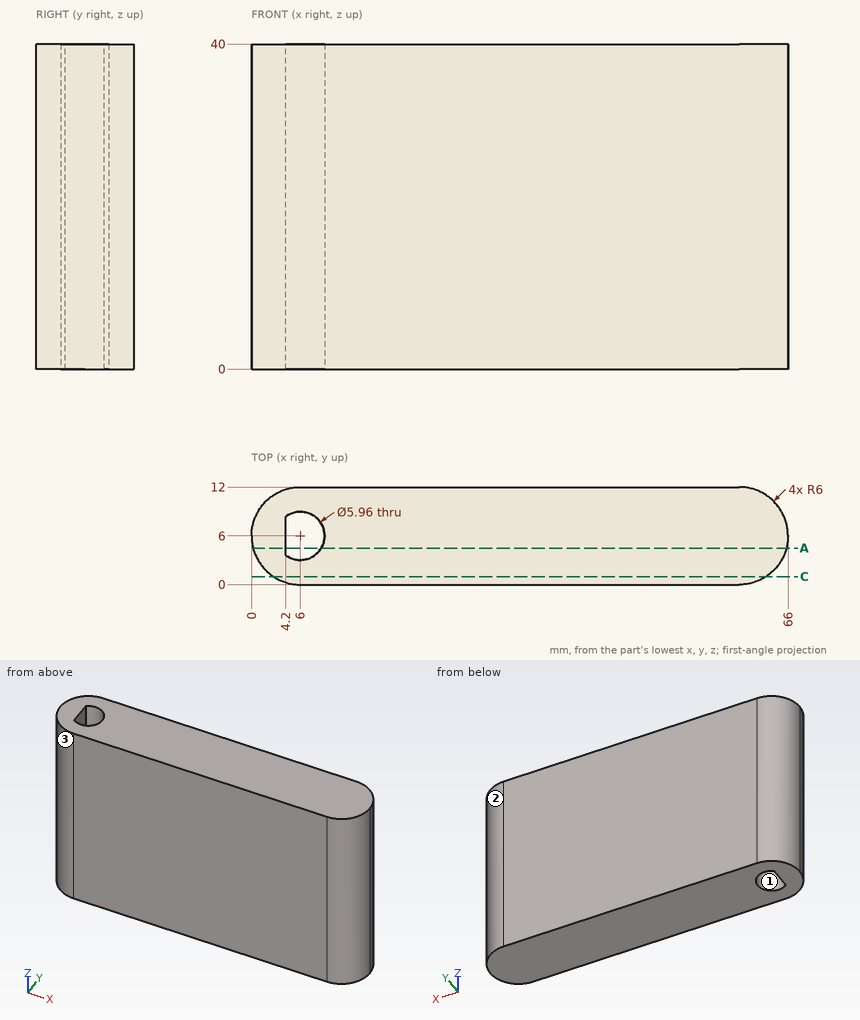
Input: dimensioned drawing with shaded views. Units: mm. Origin: part minimum x, y, z. Give positions to 0.01 mm unless a question says otherwise; leave off trailing zeros. Write each loop counter-clockwise with the first axis right and the second up, starting at its lowest first coordinate (ties: lowest second). Pieces come first, ordered by that corner, then holes. Notation, with made-up numbers: M 18.5,75.5 L 58.5,75.5 A25 cw 58.5,113.5 Z; hole C 89,-22.5 d9. An arc over 180 degrees is marked long. Return JSON: item names as keys, results as strings. Group by question number.
1) Pull-direction query (Y, two-part tool) for the marked faces 1, 2 and 3; classes: pulls with the +Y half, pulls with the -Y half, needs draft (parallel to the pull), parting line crosses it, or undercut.
2) Material intervals for line 1 along X through (y, z) = (6, 28); line 2 along Y through (x, z) = (6, 31.5); line 3 along X through (y, z) = (3.5, 5) (1 decimal), sorted ascending. Write a range as [from, to].
3) Cut plane C-C, the plane y = 1. Output: boundary loops of the cut face in (x, z), plus the area to 3 significant figures.
4) Cut plane A-A, the plane y = 4.5. Output: boundary loops of the cut face in (x, z) (1 decimal), plus the area to 3 significant figures.
Recorded:
{
 "1": {"face 1": "undercut", "face 2": "pulls with the +Y half", "face 3": "pulls with the -Y half"},
 "2": {"line 1": "x = [0, 4.2], [8.98, 66]", "line 2": "y = [0, 3.02], [8.98, 12]", "line 3": "x = [0.5, 4.4], [7.6, 65.5]"},
 "3": {"outline": "M 2.68,0 L 63.32,0 L 63.32,40 L 2.68,40 Z", "area": "2,430 mm²"},
 "4": {"outline": "M 0.2,0 L 4.2,0 L 4.2,40 L 0.2,40 Z; M 8.6,0 L 65.8,0 L 65.8,40 L 8.6,40 Z", "area": "2,450 mm²"}
}
